Design review of the part built by this model. Coordinates are the model's own, in mm. A direction names the side the tool comes from. Coordinates: 2 decimals unless noted, no trailing zeros. Loops run counter-clockwise (first coordinate to the right, second up) from the corner with the lowest first, then second, coordinate; pieces in that order, holes last. Notation, with made-up numbers: M 58.25,76.25 L 103.25,76.25 A17 ccw 103.25,107.25 Z; hole C 37,-5 d1. An arc over 180 degrees is marked long. Answer as CSV lines item,"result". Start each with the question number.
from build123d import *

# Parameters (mm, degrees)
F0_W      = 20
F0_H      = 20
F1_DEPTH  = 20
F2_R      = 3.57
F3_DEPTH  = 20.001
F5_R      = 5.5
F6_DEPTH  = 16.5
F8_DEPTH  = 20.001
F10_R     = 5.5
F11_DEPTH = 16.5
F13_DEPTH = 12.5


with BuildPart() as f1:
    # F0 (on Top) → F1 (new body)
    with BuildSketch(Plane.XY):
        Rectangle(F0_W, F0_H)
    extrude(amount=F1_DEPTH)

    # F2 (on Top) → F3 (cut, through all)
    with BuildSketch(Plane.XY):
        Circle(F2_R)
    extrude(amount=F3_DEPTH, mode=Mode.SUBTRACT)

    # F5 (on offset) → F6 (cut, through all)
    with BuildSketch(Plane.XY.offset(3.5)):
        Circle(F5_R)
    extrude(amount=F6_DEPTH, mode=Mode.SUBTRACT)

    # F7 (on face) → F8 (cut, through all)
    with BuildSketch(Plane(origin=(0, 10, 0), x_dir=(-1, 0, 0), z_dir=(0, 1, 0))):
        with BuildLine():
            Line((2.5, 9.25), (2.5, 10.75))
            ThreePointArc((2.5, 10.75), (0, 13.25), (-2.5, 10.75))
            Line((-2.5, 10.75), (-2.5, 9.25))
            ThreePointArc((-2.5, 9.25), (0, 6.75), (2.5, 9.25))
        make_face()
    extrude(amount=-F8_DEPTH, mode=Mode.SUBTRACT)

    # F10 (on offset) → F11 (cut, through all)
    with BuildSketch(Plane(origin=(0, 6.5, 0), x_dir=(-1, 0, 0), z_dir=(0, 1, 0))):
        with Locations((0, 10)):
            Circle(F10_R)
    extrude(amount=-F11_DEPTH, mode=Mode.SUBTRACT)

    # F12 (on Right) → F13 (cut, symmetric)
    with BuildSketch(Plane.YZ):
        Polygon((-10, 20), (-10, 1), (9, 20), align=None)
    extrude(amount=F13_DEPTH, both=True, mode=Mode.SUBTRACT)


solid = f1.part
Item 1: Add section D-D (y = -1.75). Give the boundary of the cut face in (x, z), plus the area to 3 significant figures.
Item 2: For pin 1 (3 mm diameter, centred on x = -2.5, y = 4, fed in from -Z); pin 2 (3.5 mm diameter, centred on x = -1, z = 11, fed in from -Y); pin 3 (9 mm diameter, centred on x = 0, y = 0, fed in from +Z), all flat-tipped, find the tip position at first contact; note any pin that passes through.
Item 3: For line 1 along X through (y, z) = (8.5, 10.75); line 2 along X through (y, z) = (0, 2.8); line 3 along Y through (x, z) = (0, 2.25), list the stretches that pass through material, from the lowest coordinate up. Write a range as from..to.
Item 4: For faces 1 (the face through (4.05, 4.74, 13.72)), 2 (the face through (-0.1, 9.5, 20)), 3 (the face through (-4.05, 3.72, 5.26)), 4 (the face through (0.05, 8.27, 6.75)), list the 3-axis set-ups (+Z, -Z, +X, -X, +Y, -Y) from which the entire face can be reached by the end or side of a thin tool; tool diameter is ignored.
Item 5: Add section B-B (z = 2.75). Give the boundary of the cut face in (x, y), plus the area to 3 significant figures.
Item 6: Mouldability with a two-part tool opening along Z and no side actions: class faces 5 (the face through (7, -1, 10)), 6 (the face through (3.405, 1.072, 1.726)), 7 (the face through (3, 6.5, 10)) as released by +Z, released by -Z, zero draft, split by the parting line, or undercut.
Item 7: Add section C-C (y = 6). Give the boundary of the cut face in (x, z).
Item 8: Add section A-A (x = 0). Give the boundary of the cut face in (y, z).
Response:
1,outline,"M -10,0 L -3.11,0 L -3.11,3.5 L -5.21,3.5 L -5.21,8.25 A5.5 cw -5.45,9.25 L -10,9.25 Z; M 3.11,0 L 10,0 L 10,9.25 L 5.45,9.25 A5.5 cw 5.21,8.25 L 5.21,3.5 L 3.11,3.5 Z"
1,area,"103 mm²"
2,pin 1,"z = 0"
2,pin 2,"y = 6.5"
2,pin 3,"z = 3.5"
3,line 1,"-10..-2.5, 2.5..10"
3,line 2,"-10..-3.57, 3.57..10"
3,line 3,"-8.75..-3.57, 3.57..10"
4,face 1,"-Y"
4,face 2,"+Z, +X, -X, +Y, -Y"
4,face 3,"+Z"
4,face 4,"+Y, -Y"
5,outline,"M -10,-8.25 L 10,-8.25 L 10,10 L -10,10 Z; hole C 0,0 d7.14"
5,area,"325 mm²"
6,face 5,"released by +Z"
6,face 6,"zero draft"
6,face 7,"undercut"
7,outline,"M -10,0 L 10,0 L 10,17 L -10,17 Z; hole C 0,10 d11"
8,outline,"M -10,0 L -3.57,0 L -3.57,3.5 L -5.5,3.5 L -5.5,4.5 L -6.5,4.5 L -10,1 Z; M 3.57,0 L 10,0 L 10,6.75 L 6.5,6.75 L 6.5,4.5 L 5.5,4.5 L 5.5,3.5 L 3.57,3.5 Z; M 5.5,15.5 L 6.5,15.5 L 6.5,13.25 L 10,13.25 L 10,20 L 9,20 L 5.5,16.5 Z"
